Build history of the part. All positions in model axes, mm. Face numbers are marked on the shaded views. A direction names the side the tool comes from. Coordinates: 2 decimals unless noted, no trailing zeros. Loops run counter-clockwise (first coordinate to the right, second up) from the corner with the lowest first, then second, coordinate; pieces in that order, holes last.
Item 1: Cut at A-A (z = 7.5). List the corners of the cut face in (x, y).
Item 2: 3-axis set-ups, long thin cutter, end or side, ignore diameter. For the marked faces 1, 2 and 3: which of +Z, -Z, +X, -X, +Y, -Y reach the whole face in a straight line?
Item 3: Cut at C-C (y = 2.25). List the corners of the cut face in (x, z).
Item 4: Flat gauge pins, fed straight in: pin 1 (10 mm diameter, centred on x = 2.5, z = -12.5, fed in from -Y); pin 2 (1.5 mm diameter, centred on x = 3, y = 12.5, fed in from -Z); pin 3 (5.5 mm diameter, centred on x = 10, z = 7.5, fed in from +Y). Where does each tip first touch, or does it go through?
Item 5: Cut at D-D (x = 14.25). List the corners of the cut face in (y, z).
Item 6: Mould opens along Z. For the marked faces 4, 5 and 6 say: released by +Z, released by -Z, zero draft, split by the parting line, or undercut.
Item 7: Cut at B-B (x = 10). List the corners of the cut face in (y, z), and give its area (4 significant figures).
Item 8: Drill centre lines: line 1 along Z through (x, y) = (10, 1.5); line 2 along Z through (x, y) = (10, 17.7); line 3 along Z through (x, y) = (1.75, 16.5). Where is each one in solid material? Low to high.
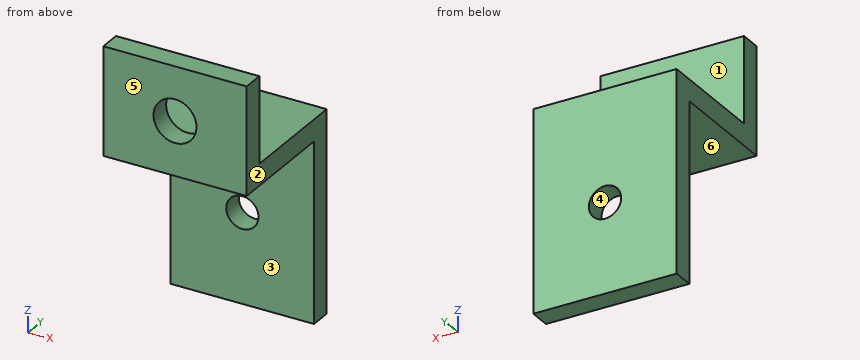
from build123d import *

# Parameters (mm, degrees)
F1_DEPTH = 20
F4_D     = 6
F5_D     = 4.5


with BuildPart() as f1:
    # F0 (on Right) → F1 (new body)
    with BuildSketch(Plane.YZ):
        Polygon((0, 15), (0, 0), (16, 0), (16, -25), (19, -25), (19, 3), (3, 3), (3, 15), align=None)
    extrude(amount=F1_DEPTH)

    # F4 (through all)
    with Locations(Plane.XZ):
        with Locations((10, 7.5)):
            Hole(F4_D / 2)

    # F5 (through all)
    with Locations(Plane.XZ.offset(-16)):
        with Locations((10, -12.5)):
            Hole(F5_D / 2)


solid = f1.part
Filled sheet:
1. outline: (0, 0) - (7, 0) - (7, 3) - (0, 3) - close; (13, 0) - (20, 0) - (20, 3) - (13, 3) - close
2. face 1: +Z, +X, -X, +Y
2. face 2: +Z, -Z, +X, +Y, -Y
2. face 3: -Z, +X, -X, -Y
3. outline: (0, 0) - (20, 0) - (20, 15) - (0, 15) - close; hole circle Ø6 at (10, 7.5)
4. pin 1: stops at y = 16
4. pin 2: stops at z = 0
4. pin 3: passes through
5. outline: (0, 0) - (16, 0) - (16, -25) - (19, -25) - (19, 3) - (3, 3) - (3, 15) - (0, 15) - close
6. face 4: undercut
6. face 5: zero draft
6. face 6: released by -Z
7. outline: (0, 0) - (16, 0) - (16, -10.25) - (19, -10.25) - (19, 3) - (3, 3) - (3, 4.5) - (0, 4.5) - close; (0, 10.5) - (3, 10.5) - (3, 15) - (0, 15) - close; (16, -25) - (19, -25) - (19, -14.75) - (16, -14.75) - close
7. area: 136.5 mm2
8. line 1: z = 0 to 4.5, 10.5 to 15
8. line 2: z = -25 to -14.75, -10.25 to 3
8. line 3: z = -25 to 3
